Work out the finished part from the listing and answer in its coordinate system (mm). A direction names the side the tool comes from. Give positions to 0.01 mm unless a question says otherwise; leave off trailing zeros. Order: outer loops, then holes, each group sorted by start corner. A loop starts at its lowest first (then second) coordinate and runs counter-clockwise, first axis right, second up. Notation, with made-up numbers: M 36,-7 L 91,-7 A15 cw 91,0 Z; hole C 50.5,78 d7. An arc over 180 degrees is marked long. One line per item, written item: value.
Autodesk Inventor part; units mm, degrees
ref_plane "YZ Plane" through (0, 0, 0) normal (1, 0, 0) x (0, 1, 0)
ref_plane "XZ Plane" through (0, 0, 0) normal (0, 1, 0) x (-1, 0, 0)
ref_plane "XY Plane" through (0, 0, 0) normal (0, 0, 1) x (1, 0, 0)
sketch "Sketch1" plane through (0, 0, 0) normal (0, 0, 1) x (1, 0, 0)
  line L0 (12.6328, -6.7) -> (10.0681, -1.2)
  line L1 (-0.0672, -6.7) -> (2.4975, -1.2)
  line L2 (-0.0672, -6.7) -> (12.6328, -6.7)
  line L3 (10.0681, 0.8) -> (2.4975, 0.8)
  line L4 (2.4975, -1.2) -> (2.4975, 0.8)
  line L5 (10.0681, -1.2) -> (10.0681, 0.8)
  line L6 (2.6975, 0.6) -> (9.8681, 0.6)
  line L7 (9.8681, 0.6) -> (9.8681, -1.2443)
  line L8 (9.8681, -1.2443) -> (12.3189, -6.5)
  line L9 (12.3189, -6.5) -> (0.2468, -6.5)
  line L10 (0.2468, -6.5) -> (2.6975, -1.2443)
  line L11 (2.6975, -1.2443) -> (2.6975, 0.6)
  line L12 (6.2828, 2.7247) -> (6.2828, -9.3147) construction
  point P0 (0, 0)
  point P1 (19.05, 0)
  point P2 (0, 0)
  dimension "d20" = 12.7
  dimension "d22" = 5.5
  dimension "d23" = 5.5
  dimension "d24" = 2
  dimension "d25" = 2
  dimension "d28" = 0.2
  dimension "d29" = 155
  dimension "d31" = 155
extrude "Extrusion1" add sketch "Sketch1" along normal blind 25.4 contours L6 L7 L8 L9 L10 L11
hole "Hole1" at (6.4769, -6.5, 20.4) direction (0, 1, 0) diameter 3.6 end through all counterbore diameter 7 counterbore depth 2.6
hole "Hole2" at (6.4769, -6.5, 5) direction (0, 1, 0) diameter 3.6 end through all counterbore diameter 7 counterbore depth 2.6
properties part number "Wall_mount"
(1) Section D-D, the plane x = 9 is taken. Give the vertices of the cut face in (y, z), then the cut area to 3 significant figures.
Findings:
outline: M -6.5,0 L 0.6,0 L 0.6,25.4 L -6.5,25.4 L -6.5,22.83 L -3.9,22.83 L -3.9,17.97 L -6.5,17.97 L -6.5,7.43 L -3.9,7.43 L -3.9,2.57 L -6.5,2.57 Z
area: 155 mm^2
(2) Which of the six approach directions +Z, -Z, +X, -X, +Y, -Y give full straight-line access (tool end or side, diameter ignored) to faces 4 (the flat face through (2.698, 0, 13)), 5 (the flat face through (9.868, 0, 13)), 6 (the cylindrical face through (9.894, -5.182, 21.159))?
Findings:
face 4: +Z, -Z, -X, +Y
face 5: +Z, -Z, +X, +Y
face 6: -Y
(3) Section C-C, the plane y = -6 is taken. Give the vertices of the cut face in (x, z).
Findings:
outline: M 0.48,0 L 12.09,0 L 12.09,25.4 L 0.48,25.4 Z; hole C 6.48,5 d7; hole C 6.48,20.4 d7
(4) Given P1, Ø4.5, axis at x = 6.48, z = 20.4, coming from the -Y side; P2, Ø3, axis at y = -4, z = 16, coming from the -X side; P3, Ø2, axis at y = -0.5, z = 18, coming from the +X side; P4, Ø3, axis at x = 6.48, z = 5, coming from the -Y side, each flat-ended and moving along its own axis, determine where each tip first touches the part or whether it passes through.
Findings:
P1: stops at y = -3.9
P2: stops at x = 0.71
P3: stops at x = 9.99
P4: passes through
(5) Section B-B, the plane x = 5.25 is taken. Give the vertices of the cut face in (y, z), then the cut area to 3 significant figures.
Findings:
outline: M -6.5,0 L 0.6,0 L 0.6,3.68 L -3.9,3.68 L -3.9,1.72 L -6.5,1.72 Z; M -6.5,8.28 L -3.9,8.28 L -3.9,6.32 L 0.6,6.32 L 0.6,19.08 L -3.9,19.08 L -3.9,17.12 L -6.5,17.12 Z; M -6.5,23.68 L -3.9,23.68 L -3.9,21.72 L 0.6,21.72 L 0.6,25.4 L -6.5,25.4 Z
area: 123 mm^2
(6) Determine the mould class of faces 1 (the flat face through (8, -3.9, 19)), 2 (the flat face through (6, 0.6, 13)), 3 (the flat face through (1.455, -3.909, 12.522)) for opening direction X: pulls with the +X half, pulls with the -X half, needs draft (parallel to the pull), parting line crosses it, or undercut.
Findings:
face 1: undercut
face 2: needs draft
face 3: pulls with the -X half
(7) Find the intervals of material crossed by probe 1 along X at (y, z) = (-1.25, 5); probe 2 along Z at (x, y) = (5, -0.75); probe 3 along Z at (x, y) = (9.25, -5.5), in increasing order. Write a range as from..to.
Findings:
probe 1: x = 2.69..4.68, 8.28..9.87
probe 2: z = 0..3.97, 6.03..19.37, 21.43..25.4
probe 3: z = 0..2.86, 7.14..18.26, 22.54..25.4
(8) Section A-A, the plane z = 20.4 is taken. Give the vertices of the cut face in (x, y), then the cut area to 3 significant figures.
Findings:
outline: M 0.25,-6.5 L 2.98,-6.5 L 2.98,-3.9 L 4.68,-3.9 L 4.68,0.6 L 2.7,0.6 L 2.7,-1.24 Z; M 8.28,-3.9 L 9.98,-3.9 L 9.98,-6.5 L 12.32,-6.5 L 9.87,-1.24 L 9.87,0.6 L 8.28,0.6 Z
area: 29.4 mm^2
